Autodesk Inventor part; units mm, degrees
ref_plane "YZ Plane" through (0, 0, 0) normal (1, 0, 0) x (0, 1, 0)
ref_plane "XZ Plane" through (0, 0, 0) normal (0, 1, 0) x (-1, 0, 0)
ref_plane "XY Plane" through (0, 0, 0) normal (0, 0, 1) x (1, 0, 0)
sketch "Sketch1" plane through (0, 0, 0) normal (0, 1, 0) x (-1, 0, 0)
  circle A0 centre (0, 0) radius 29.21
  dimension "d0" = 58.42
extrude "Extrusion1" add sketch "Sketch1" along normal blind 5.588
sketch "Sketch2" plane through (0, 5.588, 0) normal (0, 1, 0) x (1, 0, 0)
  line L0 (0, 0) -> (0, -10.16)
  line L1 (0, -10.16) -> (-2.54, -10.16)
  line L2 (-2.54, -10.16) -> (2.54, -10.16)
  line L3 (2.54, -10.16) -> (2.54, 10.16)
  line L4 (2.54, 10.16) -> (-2.54, 10.16)
  line L5 (-2.54, 10.16) -> (-2.54, -10.16)
  dimension "d3" = 10.16
  dimension "d4" = 2.54
  dimension "d5" = 5.08
  dimension "d6" = 20.32
extrude "Extrusion2" cut sketch "Sketch2" against normal blind 5.588
properties part number "open4" material "Plastic, Transparent"
CAD build for the part. Positions are in the model's coordinates, mm. A direction names the side the tool comes from. Round coordinates to 2 decimals unless told otherwise and drop trailing zeros. Order: outer loops, then holes, each group sorted by start corner. A loop starts at its lowest first (then second) coordinate and runs counter-clockwise, first axis right, second up.
Item 1: Saw through at A-A on x = 0. Write the cut outline in (y, z).
Item 2: Tool access for faces 1 (the face through (0, 3, 10.16)), 2 (the face through (-6, 5.588, 0)): list every direction of +Z, -Z, +X, -X, +Y, -Y with a clear straight run to the whole face (end or side of a thin tool).
Item 3: Saw through at D-D on x = 12. Write the cut outline in (y, z), then the cut area to 3 significant figures.
Item 4: Pin check, flat tips, straight feed: pin 1 (1.5 mm diameter, centred on x = -1, y = 2.5, fed in from -Z); pin 2 (2 mm diameter, centred on x = -8.5, y = 5, fed in from -Z); pin 3 (1.5 mm diameter, centred on x = -18.5, y = 4.5, fed in from -Z). Stop position of each tip, or through.
Item 5: Saw through at B-B on z = 0. Write the cut outline in (x, y), then the cut area to 3 significant figures.
Item 6: Probe line 1 along X through (y, z) = (2.9, -0.5); line 2 along Z through (x, y) = (-2, 4.35); line 3 along X through (y, z) = (2.6, -5). List the from-to ranges inside material, lowest first.
Item 7: Saw through at C-C on y = 3.55. Write the cut outline in (x, z), then the cut area to 3 significant figures.
Reported:
1. outline: (0, -29.21) - (5.59, -29.21) - (5.59, -10.16) - (0, -10.16) - close; (0, 10.16) - (5.59, 10.16) - (5.59, 29.21) - (0, 29.21) - close
2. face 1: +Y, -Y
2. face 2: +Z, -Z, +X, -X, +Y
3. outline: (0, -26.63) - (5.59, -26.63) - (5.59, 26.63) - (0, 26.63) - close
3. area: 298 mm2
4. pin 1: stops at z = -29.21
4. pin 2: stops at z = -28.23
4. pin 3: stops at z = -23.2
5. outline: (-29.21, 0) - (-2.54, 0) - (-2.54, 5.59) - (-29.21, 5.59) - close; (2.54, 0) - (29.21, 0) - (29.21, 5.59) - (2.54, 5.59) - close
5. area: 298 mm2
6. line 1: x = -29.21 to -2.54, 2.54 to 29.21
6. line 2: z = -29.14 to -10.16, 10.16 to 29.14
6. line 3: x = -28.78 to -2.54, 2.54 to 28.78
7. outline: circle Ø58.42 at (0, 0); hole (-2.54, -10.16) - (2.54, -10.16) - (2.54, 10.16) - (-2.54, 10.16) - close
7. area: 2,580 mm2
